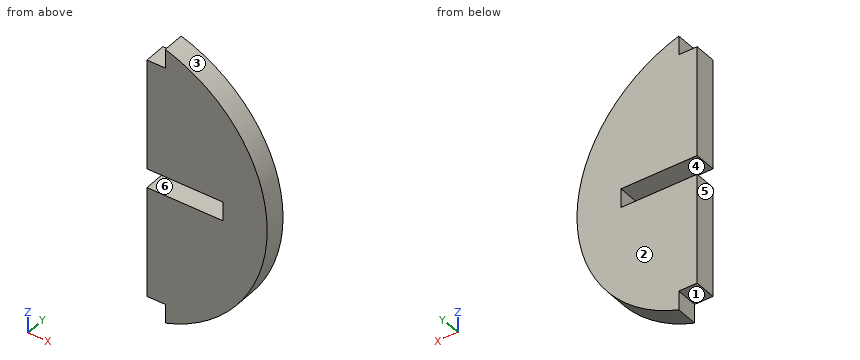
from build123d import *

# Parameters (mm, degrees)
BOSS_EXTRUDE1_DEPTH      = 1.5
BOSS_EXTRUDE1_DEPTH_BACK = 1.5


with BuildPart() as part:
    # Sketch1 → Boss-Extrude1 (new, two sides: drawn at the far end of the back side and taken through both)
    with BuildSketch(Plane(origin=(0, 0, 0), x_dir=(1, 0, 0), z_dir=(0, 1, 0)).offset(-BOSS_EXTRUDE1_DEPTH_BACK)):
        with BuildLine():
            Line((3.621320344, -1.3), (14, -1.3))
            Line((14, -1.3), (14, 1.3))
            Line((14, 1.3), (3.621320344, 1.3))
            Line((3.621320344, 1.3), (3.621320344, 16.440205809))
            Line((3.621320344, 16.440205809), (6.121320344, 16.440205809))
            Line((6.121320344, 16.440205809), (6.121320344, 19.040205809))
            ThreePointArc((6.121320344, 19.040205809), (20, 0), (6.121320344, -19.040205809))
            Line((6.121320344, -19.040205809), (6.121320344, -16.440205809))
            Line((6.121320344, -16.440205809), (3.621320344, -16.440205809))
            Line((3.621320344, -16.440205809), (3.621320344, -1.3))
        make_face()
    extrude(amount=BOSS_EXTRUDE1_DEPTH + BOSS_EXTRUDE1_DEPTH_BACK)


solid = part.part
Model file for the job. Use its own axes, mm. Face numbers are marked on the shaded views. A direction names the side the tool comes from. Round coordinates to 2 decimals unless told otherwise and drop trailing zeros. Loops run counter-clockwise (first coordinate to the right, second up) from the corner with the lowest first, then second, coordinate; pieces in that order, holes last. Notation, with made-up numbers: M 85,7.25 L 143,7.25 A26 ccw 143,46.25 Z; hole C 42.25,80.25 d11. An arc over 180 degrees is marked long. One line per question, with ' | ' between items.
1) Mould opens along Z. For the marked faces 3, 4, 5 and 6 say: +Z half, -Z half, draft (parallel to the pull), parting line (faces both ways), or undercut.
Solved:
face 3: parting line | face 4: undercut | face 5: draft | face 6: undercut
2) Band-saw the part on D-D (x = 13). Give the cut face in (y, z), then the cut area to 3 significant figures.
Solved:
outline: M -1.5,-15.2 L 1.5,-15.2 L 1.5,-1.3 L -1.5,-1.3 Z; M -1.5,1.3 L 1.5,1.3 L 1.5,15.2 L -1.5,15.2 Z | area: 83.4 mm²
3) Band-saw the part on A-A (x = 5.75). Give the cut face in (y, z).
Solved:
outline: M -1.5,-16.44 L 1.5,-16.44 L 1.5,-1.3 L -1.5,-1.3 Z; M -1.5,1.3 L 1.5,1.3 L 1.5,16.44 L -1.5,16.44 Z
4) Band-saw the part on B-B (y = -0.5). Give the cut face in (x, z).
Solved:
outline: M 3.62,-16.44 L 6.12,-16.44 L 6.12,-19.04 A20 ccw 6.12,19.04 L 6.12,16.44 L 3.62,16.44 L 3.62,1.3 L 14,1.3 L 14,-1.3 L 3.62,-1.3 Z
5) Flat gauge pin, fed straight in: pin 1 (0.8 mm diameter, centred on x = 5, y = 0, fed in from +Z). Where does the tip first touch, or does it go through?
Solved:
pin 1: stops at z = 16.44
6) Band-saw the part on C-C (z = 0). Give the cut face in (x, y), then the cut area to 3 significant figures.
Solved:
outline: M 14,-1.5 L 20,-1.5 L 20,1.5 L 14,1.5 Z | area: 18.0 mm²
7) Drill centre lines: line 1 along Z through (x, y) = (10.5, -1.4); line 2 along Z through (x, y) = (4.75, -1.05); line 3 along X through (y, z) = (0.6, 0). Where is each one in solid material? Low to high.
Solved:
line 1: z = -17.02 to -1.3, 1.3 to 17.02 | line 2: z = -16.44 to -1.3, 1.3 to 16.44 | line 3: x = 14 to 20
8) 3-axis set-ups, long thin cutter, end or side, ignore diameter. For the marked faces 1 and 2: which of +Z, -Z, +X, -X, +Y, -Y reach the whole face in a straight line?
Solved:
face 1: -Z, -X, +Y, -Y | face 2: +Z, -Z, +X, -X, +Y
